```python
from build123d import *

# Parameters (mm, degrees)
SKETCH3_R           = 43.0784
SKETCH3_R_2         = 39.9034
BOSS_EXTRUDE1_DEPTH = 3.175
SKETCH4_R           = 0.79375
CUT_EXTRUDE1_DEPTH  = 62.004735211
CIRPATTERN1_COUNT   = 4


with BuildPart() as part:
    # Sketch3 → Boss-Extrude1 (new, symmetric)
    with BuildSketch(Plane.XY):
        Circle(SKETCH3_R)
        Circle(SKETCH3_R_2, mode=Mode.SUBTRACT)
    extrude(amount=BOSS_EXTRUDE1_DEPTH, both=True)

    # Sketch4 → Cut-Extrude1 (cut, through all)
    with BuildSketch(Plane(origin=(0, 0, 0), x_dir=(1, 0, 0), z_dir=(0, 1, 0))):
        with Locations(Location((0, 0, 0), (0, 0, 270))):
            Circle(SKETCH4_R)
    cut_extrude1 = extrude(amount=-CUT_EXTRUDE1_DEPTH, mode=Mode.SUBTRACT)

    # CirPattern1: Cut-Extrude1 ×4 about axis
    cirpattern1_axis = Axis((0, 0, 3.175), (0, 0, -1))
    for i in range(1, CIRPATTERN1_COUNT):
        add(cut_extrude1.rotate(cirpattern1_axis, i * 360 / CIRPATTERN1_COUNT), mode=Mode.SUBTRACT)


solid = part.part
```
Verification items for the finished model (mm, model axes). Coordinates: 2 decimals unless noted, no trailing zeros. Write each loop counter-clockwise with the first axis right and the second up, starting at its lowest first coordinate (ties: lowest second). Pieces come first, ordered by that corner, then holes. Notation, with made-up numbers: M 72,51.5 L 108,51.5 A27 cw 108,76.5 Z; hole C 9.25,35 d3. An arc over 180 degrees is marked long. One line per item, written item: value.
Item 1: Section check A-A, the plane x = 32.5. Record the boundary of the cut face in (y, z) (3 decimals).
Check sheet entries:
outline: M -28.275,-3.175 L -23.152,-3.175 L -23.152,3.175 L -28.275,3.175 Z; M 23.152,-3.175 L 28.275,-3.175 L 28.275,3.175 L 23.152,3.175 Z
Item 2: Mould release check, pull along X, two halves, no side actions. Record for faces 1 (the cylindrical face through (-9.339, -42.054, 0.044)), 2 (the cylindrical face through (38.06, 11.99, -0.04)), 3 (the flat face through (13, -38, 3.175)): pulls with the +X half, pulls with the -X half, needs draft (parallel to the pull), parting line crosses it, or undercut.
Check sheet entries:
face 1: parting line crosses it
face 2: undercut
face 3: needs draft
Item 3: Section check B-B, the plane y = -36. Record the boundary of the cut face in (x, z) (3 decimals).
Check sheet entries:
outline: M -23.659,-3.175 L -17.213,-3.175 L -17.213,3.175 L -23.659,3.175 Z; M 17.213,-3.175 L 23.659,-3.175 L 23.659,3.175 L 17.213,3.175 Z
Item 4: Scan lines: line 1 along X through (y, z) = (0, 1.25); line 2 along Z through (x, y) = (0, -40.6) (3 decimals); line 3 along Y through (x, z) = (1, 2.75). Record each from-to range of solid material in increasing order.
Check sheet entries:
line 1: x = -43.08 to -39.9, 39.9 to 43.08
line 2: z = -3.175 to -0.794, 0.794 to 3.175
line 3: y = -43.07 to -39.89, 39.89 to 43.07
Item 5: Gauge pin test, flat ends, axial feed: pin 1 Ø1.5 at (x, z) = (-14.5, -1.5) entering from -Y; pin 2 Ø1 at (x, z) = (21.5, -1) entering from +Y. Record the tip position at first contact, or that the pin passes through.
Check sheet entries:
pin 1: stops at y = -40.83
pin 2: stops at y = 37.61
Item 6: Section check C-C, the plane z = 2. Record the boundary of the cut face in (x, y), plus the area to 3 significant figures.
Check sheet entries:
outline: C 0,0 d86.16; hole C 0,0 d79.81
area: 828 mm^2
